Autodesk Inventor part; units mm, degrees
ref_plane "YZ Plane" through (0, 0, 0) normal (1, 0, 0) x (0, 1, 0)
ref_plane "XZ Plane" through (0, 0, 0) normal (0, 1, 0) x (-1, 0, 0)
ref_plane "XY Plane" through (0, 0, 0) normal (0, 0, 1) x (1, 0, 0)
sketch "Sketch1" plane through (0, 0, 0) normal (0, 1, 0) x (-1, 0, 0)
  circle A0 centre (0, 0) radius 4.0309
  circle A1 centre (0, 0) radius 3.3
  dimension "d0" = 6.6
extrude "Extrusion1" add sketch "Sketch1" along normal blind 42
sketch "Sketch2" plane through (0, 42, 0) normal (0, 1, 0) x (1, 0, 0)
  circle A0 centre (0, 0) radius 4.0309
  circle A1 centre (0, 0) radius 3.3
  circle A2 centre (0, 0) radius 2.8
  dimension "d3" = 5.6
extrude "Extrusion2" add sketch "Sketch2" against normal blind 5 contours A1
sketch "Sketch3" plane through (0, 42, 0) normal (0, 1, 0) x (1, 0, 0)
  circle A0 centre (0, 0) radius 38.5
  circle A1 centre (0, 0) radius 25
  circle A2 centre (0, 0) radius 4.0309
  circle A3 centre (0, 0) radius 2.8
  line L0 (0, 4.0309) -> (38.2884, 4.0309)
  line L1 (0, -4.0309) -> (38.2884, -4.0309)
  line L2 (-3.4908, -2.0154) -> (-22.635, 31.1433)
  line L3 (3.4908, 2.0154) -> (-15.6534, 35.1742)
  line L4 (3.4908, -2.0154) -> (-15.6534, -35.1742)
  line L5 (-3.4908, 2.0154) -> (-22.635, -31.1433)
  point P0 (24.6729, 4.0309)
  point P1 (24.6729, -4.0309)
  point P2 (-4.6544, 0)
  point P3 (-3.4908, 2.0154)
  point P4 (2.3272, 4.0309)
  point P5 (-8.8456, 23.3828)
  point P6 (-15.8273, 19.3519)
  point P7 (-15.8273, -19.3519)
  point P8 (-8.8456, -23.3828)
  point P9 (2.3272, -4.0309)
  point P10 (-3.4908, -2.0154)
  point P11 (-22.635, -31.1433)
  point P12 (-22.635, 31.1433)
  point P13 (3.4908, -2.0154)
  point P14 (-15.6534, -35.1742)
  point P15 (-15.6534, 35.1742)
  dimension "d10" = 77
  dimension "d11" = 50
  dimension "d28" = 360
extrude "Extrusion3" add sketch "Sketch3" against normal blind 0.6 contours A0 L1 A1 L0 | L0 A1 L3 A0 | A0 L4 A1 L1 | L3 A1 L2 A0 | L0 L3 A1 | A1 L1 L4 A2 L3 L0 | A0 L5 A1 L4 | A1 L4 L1 | L2 A1 L5 A0 | L3 L0 A2 L5 L2 A1 | L3 A2 L0 | A1 L5 L2 A2 L1 L4 | L1 A2 L4 | L2 L5 A1 | A2 | L5 A2 L2 | A3
fillet "Fillet1" [suppressed]
sketch "Sketch4" plane through (0, 42, 0) normal (0, 1, 0) x (1, 0, 0)
  circle A0 centre (0, 0) radius 39.5
  circle A1 centre (0, 0) radius 37.5
  circle A2 centre (0, 0) radius 29.5
  line L0 (-39.5, 0) -> (0, 0)
  line L1 (0, 0) -> (-37.3194, 3.6756)
  line L2 (0, 0) -> (-37.3194, -3.6756)
  line L3 (0, 0) -> (-35.8853, -10.8857)
  line L4 (0, 0) -> (-33.072, -17.6774)
  line L5 (0, 0) -> (-28.9879, -23.7897)
  line L6 (0, 0) -> (-23.7897, -28.9879)
  line L7 (0, 0) -> (-17.6774, -33.072)
  line L8 (0, 0) -> (-10.8857, -35.8853)
  line L9 (0, 0) -> (-3.6756, -37.3194)
  line L10 (0, 0) -> (3.6756, -37.3194)
  line L11 (0, 0) -> (10.8857, -35.8853)
  line L12 (0, 0) -> (17.6774, -33.072)
  line L13 (0, 0) -> (23.7897, -28.9879)
  line L14 (0, 0) -> (28.9879, -23.7897)
  line L15 (0, 0) -> (33.072, -17.6774)
  line L16 (0, 0) -> (35.8853, -10.8857)
  line L17 (0, 0) -> (37.3194, -3.6756)
  line L18 (0, 0) -> (37.3194, 3.6756)
  line L19 (0, 0) -> (35.8853, 10.8857)
  line L20 (0, 0) -> (33.072, 17.6774)
  line L21 (0, 0) -> (28.9879, 23.7897)
  line L22 (0, 0) -> (23.7897, 28.9879)
  line L23 (0, 0) -> (17.6774, 33.072)
  line L24 (0, 0) -> (10.8857, 35.8853)
  line L25 (0, 0) -> (3.6756, 37.3194)
  line L26 (0, 0) -> (-3.6756, 37.3194)
  line L27 (0, 0) -> (-10.8857, 35.8853)
  line L28 (0, 0) -> (-17.6774, 33.072)
  line L29 (0, 0) -> (-23.7897, 28.9879)
  line L30 (0, 0) -> (-28.9879, 23.7897)
  line L31 (0, 0) -> (-33.072, 17.6774)
  line L32 (0, 0) -> (-35.8853, 10.8857)
  point P0 (-23.7897, -28.9879)
  point P1 (-18.7146, -22.8038)
  point P2 (-22.8038, -18.7146)
  point P3 (-28.9879, -23.7897)
  point P4 (-10.8857, -35.8853)
  point P5 (-8.5634, -28.2297)
  point P6 (-13.9062, -26.0167)
  point P7 (-17.6774, -33.072)
  point P8 (3.6756, -37.3194)
  point P9 (2.8915, -29.3579)
  point P10 (-2.8915, -29.3579)
  point P11 (17.6774, -33.072)
  point P12 (13.9062, -26.0167)
  point P13 (8.5634, -28.2297)
  point P14 (10.8857, -35.8853)
  point P15 (28.9879, -23.7897)
  point P16 (22.8038, -18.7146)
  point P17 (18.7146, -22.8038)
  point P18 (23.7897, -28.9879)
  point P19 (35.8853, -10.8857)
  point P20 (28.2297, -8.5634)
  point P21 (26.0167, -13.9062)
  point P22 (33.072, -17.6774)
  point P23 (-33.072, -17.6774)
  point P24 (-26.0167, -13.9062)
  point P25 (-28.2297, -8.5634)
  point P26 (-35.8853, -10.8857)
  point P27 (-29.3579, -2.8915)
  point P28 (-29.3579, 2.8915)
  point P29 (37.3194, 3.6756)
  point P30 (29.3579, 2.8915)
  point P31 (29.3579, -2.8915)
  point P32 (37.3194, -3.6756)
  point P33 (33.072, 17.6774)
  point P34 (26.0167, 13.9062)
  point P35 (28.2297, 8.5634)
  point P36 (35.8853, 10.8857)
  point P37 (23.7897, 28.9879)
  point P38 (18.7146, 22.8038)
  point P39 (22.8038, 18.7146)
  point P40 (28.9879, 23.7897)
  point P41 (10.8857, 35.8853)
  point P42 (8.5634, 28.2297)
  point P43 (13.9062, 26.0167)
  point P44 (17.6774, 33.072)
  point P45 (-3.6756, 37.3194)
  point P46 (-2.8915, 29.3579)
  point P47 (2.8915, 29.3579)
  point P48 (3.6756, 37.3194)
  point P49 (-17.6774, 33.072)
  point P50 (-13.9062, 26.0167)
  point P51 (-8.5634, 28.2297)
  point P52 (-10.8857, 35.8853)
  point P53 (-35.8853, 10.8857)
  point P54 (-28.2297, 8.5634)
  point P55 (-26.0167, 13.9062)
  point P56 (-33.072, 17.6774)
  point P57 (-28.9879, 23.7897)
  point P58 (-22.8038, 18.7146)
  point P59 (-18.7146, 22.8038)
  point P60 (-23.7897, 28.9879)
  dimension "d15" = 2
  dimension "d16" = 8
  dimension "d17" = 5.625
  dimension "d19" = 5.625
  dimension "d22" = 360
extrude "Extrusion4" cut sketch "Sketch4" against normal through all contours A1 L1 A2 L0 | L0 A2 L2 A1 | A1 L31 A2 L32 | L3 A2 L4 A1 | A2 L6 A1 L5 | A2 L8 A1 L7 | A2 L10 A1 L9 | A2 L12 A1 L11 | A2 L14 A1 L13 | A2 L16 A1 L15 | A2 L18 A1 L17 | A2 L20 A1 L19 | A2 L22 A1 L21 | A2 L24 A1 L23 | A2 L26 A1 L25 | A2 L28 A1 L27 | A2 L30 A1 L29
fillet "Fillet2" [suppressed]
sketch "Sketch5" plane through (0, 41.4, 0) normal (0, -1, 0) x (1, 0, 0)
  circle A0 centre (0, 0) radius 2.8
extrude "Extrusion5" cut sketch "Sketch5" against normal blind 0.6
fillet "Fillet3" radius 2 1 edges at (4.0309, 41.4, 0)
sketch "Sketch6" plane through (0, 41.4, 0) normal (0, -1, 0) x (1, 0, 0)
  circle A0 centre (0, 0) radius 25
  circle A1 centre (0, 0) radius 4.0309
  circle A2 centre (0, 0) radius 22.5
  dimension "d34" = 50
  dimension "d35" = 45
extrude "Extrusion6" add sketch "Sketch6" along normal blind 5 contours A0
fillet "Fillet4" radius 1 2 edges at (-22.5, 41.4, 0) (-25, 41.4, 0)
properties part number "Eje_econder" material "PET Plastic"
Here's how the part is built. I have some questions about the finished solid (model axes, mm). A direction names the side the tool comes from. Coordinates: 2 decimals unless noted, no trailing zeros. Order: outer loops, then holes, each group sorted by start corner. A loop starts at its lowest first (then second) coordinate and runs counter-clockwise, first axis right, second up. Notation, with made-up numbers: M 56,31.5 L 65,31.5 A21 cw 65,53.5 Z; hole C 70,3.25 d2. An arc over 180 degrees is marked long. Answer as a JSON object with one key per item and string values. Group by question number.
(1) Suppose I cut it at C-C, the plane y = 20. Please give me the cut outline in (x, z).
(2) Which directions (+Z, -Z, +X, -X, +Y, -Y) give clear straight access to the entire face, cutting with the end or side of a thin tool? Please do faces 1 (the face through (-3.845, 19.424, -1.211)), 2 (the face through (-25.853, 41.704, 21.217)).
(3) Suppose I cut it at A-A, the plane z = 0. State how many separate pieces and enclosed holes the cut face has, then the cut area to 3 significant figures.
(4) I need wall thicknesses on probe 1 along Z at (x, y) = (0, 38); probe 2 along Y at (x, z) = (19.5, 26); probe 3 along Z at (x, y) = (0, 40). Which ranges of each line are inside material? Lowest first, please.
(5) For pin 1 (1.5 mm diameter, centred on x = 1, y = 12, fed in from -Z); pin 2 (12 mm diameter, centred on x = 5.5, z = -15, fed in from -Y); pin 3 (1 mm diameter, centred on x = 8, z = -12, fed in from -Y), each with a flat end and sliding along its axis, tell me the tip position at first contact or that it passes through.
(6) If we mould it in two halves opening along X, with no side actions, what happens to faces 3 (the face through (21.217, 41.704, -25.853)), 4 (the face through (11.327, 41.704, -27.239)), 5 (the face through (2, 0, -3))? For each: released by +X, released by -X, zero draft, split by the parting line, or undercut.
(7) Suppose I cut it at B-B, the plane x = -31. Please give me the cut outline in (y, z), then the cut area to 3 significant figures.
Values found:
{
 "1": {"outline": "C 0,0 d8.06; hole C 0,0 d6.6"},
 "2": {"face 1": "-Y", "face 2": "+Y, -Y"},
 "3": {"separate pieces": "4", "enclosed holes": "0", "area": "126 mm^2"},
 "4": {"probe 1": "z = -25 to -22.5, -4.03 to -2.8, 2.8 to 4.03, 22.5 to 25", "probe 2": "y = 41.4 to 42", "probe 3": "z = -25 to -22.5, -4.12 to -2.8, 2.8 to 4.12, 22.5 to 25"},
 "5": {"pin 1": "stops at z = -4.02", "pin 2": "stops at y = 41.28", "pin 3": "stops at y = 41.4"},
 "6": {"face 3": "undercut", "face 4": "undercut", "face 5": "zero draft"},
 "7": {"outline": "M 41.4,-22.83 L 42,-22.83 L 42,-16.57 L 41.4,-16.57 Z; M 41.4,-9.4 L 42,-9.4 L 42,-3.05 L 41.4,-3.05 Z; M 41.4,3.05 L 42,3.05 L 42,9.4 L 41.4,9.4 Z; M 41.4,16.57 L 42,16.57 L 42,22.83 L 41.4,22.83 Z", "area": "15.1 mm^2"}
}
